Work out the finished part from the listing and answer in its coordinate system (mm). Coordinates: 2 decimals unless noted, no trailing zeros. Write each loop counter-clockwise with the first axis right and the second up, starting at its lowest first coordinate (ties: lowest second). Pieces come first, ordered by that corner, then holes. Notation, with made-up numbers: (-25.75, 35.25) - (23.25, 35.25) arc R32 cw to (23.25, 73.25) - close; hole circle Ø2 at (54.25, -2). An arc over 180 degrees is marked (long way). Use a Markdown table: item, result. Add a question column.
(1) The part is cut by section B-B, the plane y = 4.5. Give the vertices of the cut face in (x, z).
(2) Find the intervals of material crossed by line 1 (X direction, y = 0.5, z = -749.3); line 2 (X direction, y = 4.5, z = -957); line 3 (Y direction, x = -6.5, z = -159.5), in increasing order. Write a range as from..to.
(3) Given pin 1 Ø7 at (x, z) = (-11.5, -528.5) entering from +Y; pin 2 Ø4 at (x, z) = (-14.3, -66.68) entering from +Y; pin 3 Ø6 at (x, z) = (8.5, -1075.5) entering from -Y; pin 4 Ø3 at (y, z) = (5, -621) entering from +X, each flat-ended and moving along its own axis, determine where each tip first touches the part or whether it passes through.
(4) The part is cut by section A-A, the plane z = -249. Give the vertices of the cut face in (x, y) (3 decimals), then the cut area to 3 significant figures.
from build123d import *

# Parameters (mm, degrees)
EXTRUDE1_DEPTH     = 1498.6
SKETCH2_R          = 2.4257
CUT_EXTRUDE1_DEPTH = 1499.828690178
LPATTERN1_COUNT    = 11
LPATTERN1_PITCH    = 136.525


with BuildPart() as part:
    # Sketch1 → Extrude1 (new body)
    with BuildSketch(Plane.XY):
        with BuildLine():
            Line((-25.4, 0), (25.4, 0))
            Line((25.4, 0), (25.4, 1.524))
            Line((25.4, 1.524), (2.711977876, 1.524))
            ThreePointArc((2.711977876, 1.524), (0, 6.35), (-2.711977876, 1.524))
            Line((-2.711977876, 1.524), (-25.4, 1.524))
            Line((-25.4, 1.524), (-25.4, 0))
        make_face()
    extrude(amount=-EXTRUDE1_DEPTH)

    # Sketch2 → Cut-Extrude1 (cut, through all)
    with BuildSketch(Plane(origin=(0, 0, 0), x_dir=(1, 0, 0), z_dir=(0, 1, 0))):
        with Locations(Location((14.3002, 66.675, 0), (0, 0, 180))):
            Circle(SKETCH2_R)
        with Locations(Location((-14.3002, 66.675, 0), (0, 0, 180))):
            Circle(SKETCH2_R)
    cut_extrude1 = extrude(amount=CUT_EXTRUDE1_DEPTH, mode=Mode.SUBTRACT)

    # LPattern1: Cut-Extrude1 ×11
    with Locations(*[(0, 0, -i * LPATTERN1_PITCH) for i in range(1, LPATTERN1_COUNT)]):
        add(cut_extrude1, mode=Mode.SUBTRACT)


solid = part.part
Model answer:
| question | item | result |
|---|---|---|
| 1 | outline | (-2.89, -1498.6) - (2.89, -1498.6) - (2.89, 0) - (-2.89, 0) - close |
| 2 | line 1 | -25.4..-16.73, -11.87..11.87, 16.73..25.4 |
| 2 | line 2 | -2.89..2.89 |
| 2 | line 3 | 0..1.52 |
| 3 | pin 1 | y = 1.52 |
| 3 | pin 2 | through |
| 3 | pin 3 | y = 0 |
| 3 | pin 4 | x = 3.16 |
| 4 | outline | (-25.4, 0) - (25.4, 0) - (25.4, 1.524) - (2.712, 1.524) arc R3.175 ccw (long way) to (-2.712, 1.524) - (-25.4, 1.524) - close |
| 4 | area | 103 mm^2 |
